Work out the finished part from the listing and answer in its coordinate system (mm). A direction names the side the tool comes from. Round coordinates to 2 decimals unless told otherwise and drop trailing zeros. Write each loop counter-clockwise with the first axis right and the second up, starting at its lowest first coordinate (ties: lowest second). Pieces come first, ordered by that corner, then holes. Notation, with made-up numbers: (48, 32) - (80, 32) arc R17 ccw to (80, 62) - close; hole circle Ø6 at (-23.75, 85). An arc over 180 degrees is marked (long way). Write item = value, one per line. Start each with the question number.
Autodesk Inventor part; units mm, degrees
ref_plane "YZ Plane" through (0, 0, 0) normal (1, 0, 0) x (0, 1, 0)
ref_plane "XZ Plane" through (0, 0, 0) normal (0, 1, 0) x (-1, 0, 0)
ref_plane "XY Plane" through (0, 0, 0) normal (0, 0, 1) x (1, 0, 0)
sketch "Skizze1" plane through (0, 0, 0) normal (0, 0, 1) x (1, 0, 0)
  line L0 (5, 52.5) -> (-5, 52.5)
  line L1 (-5, 52.5) -> (-5, 16)
  line L2 (5, 16) -> (5, 52.5)
  arc A0 (-7.9412, 4.2353) -> (7.9412, 4.2353) centre (0, 0) ccw
  arc A1 (5, 16) -> (7.9412, 4.2353) centre (30, 16) ccw
  arc A2 (-7.9412, 4.2353) -> (-5, 16) centre (-30, 16) ccw
  line L3 (0, -25.0931) -> (0, 22.9698)
  line L4 (0, 68.0186) -> (0, -40.6118)
  point P0 (0, 0)
  point P1 (0, 0)
  point P2 (-5, 7.4833)
  point P3 (5, 7.4833)
  dimension "d1" = 18
  dimension "d4" = 25
  dimension "d7" = 0
  dimension "d8" = 52.5
  dimension "d9" = 0
  dimension "d10" = 0
  dimension "d20" = 5
  dimension "d21" = 5
extrude "Extrusion1" add sketch "Skizze1" along normal blind 10
sketch "Skizze4" plane through (0, 0, 10) normal (0, 0, 1) x (1, 0, 0)
  circle A0 centre (0, 0) radius 6.05
  dimension "d22" = 12.1
extrude "Extrusion2" cut sketch "Skizze4" against normal blind 5.6
fillet "Rundung1" radius 0.2 1 edges at (-6.05, 0, 10)
fillet "Rundung2" radius 0.2 10 edges at (5, 34.25, 10) (0, -9, 10) (-5.7464, 9.9366, 10) (-5, 34.25, 10) (5.7464, 9.9366, 10) (5, 34.25, 0) (0, -9, 0) (-5.7464, 9.9366, 0) (-5, 34.25, 0) (5.7464, 9.9366, 0)
sketch "Skizze5" plane through (0, 0, 0) normal (0, 0, -1) x (-1, 0, 0)
  circle A0 centre (0, 0) radius 1.75
  dimension "d27" = 3.5
extrude "Extrusion3" cut sketch "Skizze5" against normal up to next
fillet "Rundung3" radius 0.2 2 edges at (1.75, 0, 0) (1.75, 0, 4.4)
sketch "Skizze6" plane through (-4.8, 52.5, 0) normal (0, 1, 0) x (1, 0, 0)
  circle A0 centre (4.8, -5) radius 1.75
  line L0 (9.6, -10) -> (0, -10)
  line L1 (9.8, -0.2) -> (9.8, -9.8)
  point P0 (4.8, 0)
  dimension "d31" = 3.5
  dimension "d32" = 5
  dimension "d33" = 5
extrude "Extrusion4" cut sketch "Skizze6" against normal blind 4
sketch "Skizze7" plane through (0, 0, 0) normal (0, 0, -1) x (-1, 0, 0)
  circle A0 centre (0, 0) radius 4
  dimension "d36" = 8
extrude "Extrusion5" cut sketch "Skizze7" against normal blind 3
sketch "Skizze8" plane through (0, 0, 0) normal (0, 0, -1) x (-1, 0, 0)
  line L0 (0, -13.3377) -> (18.2323, -13.3377)
  line L1 (18.2323, -13.3377) -> (18.2323, 56.3283)
  line L2 (18.2323, 56.3283) -> (0, 56.3283)
  line L3 (0, 56.3283) -> (0, -13.3377)
  point P0 (0, 0)
extrude "Extrusion6" cut sketch "Skizze8" against normal up to next
properties part number "alternativeJoint2"
1. Find section D-D on y = 22.5. Give the vertices of the cut face in (x, z), plus the area to 3 significant figures.
2. Find section C-C on z = 5. Give the vertices of the cut face in (x, y).
3. Consider line 1 (Z direction, x = 2, y = 1); line 2 (Y direction, x = 4.25, z = 8.75); line 3 (X direction, y = 21, z = 8). Determine where each line is inside the solid, lowest interval first.
4. Which of the six approach directions +Z, -Z, +X, -X, +Y, -Y give full straight-line access (tool end or side, diameter ignored) to faces 1 (the face through (1, 48.5, 5)), 2 (the face through (3, 22, 10)), 3 (the face through (5.77, 9.85, 4.93)), 4 (the face through (6.05, -0.13, 7.14)), 5 (the face through (4, 0, 1))?
5. Each of these flat-tipped pins is pushed along its axis until it touches: pin 1 (0.5 mm diameter, centred on x = 1, z = 4.5, fed in from +Y); pin 2 (1.8 mm diameter, centred on x = 4, y = 2.5, fed in from +Z). Where does it stop, or does it pass through?
6. Find section B-B on z = 1.5. Give the vertices of the cut face in (x, y).
7. For a pull along Y with two mould halves and no side action, classify faces 6 (the face through (3, 52.5, 5)), 7 (the face through (1.75, 0.04, 3.59)), 8 (the face through (5, 34, 5)) as released by +Y, released by -Y, zero draft, split by the parting line, or undercut.
8. Find section A-A on y = 0. Give the vertices of the cut face in (x, z).
Answer key:
q1.outline = (0, 0) - (4.8, 0) arc R0.2 ccw to (5, 0.2) - (5, 9.8) arc R0.2 ccw to (4.8, 10) - (0, 10) - close
q1.area = 50.0 mm²
q2.outline = (0, -9) arc R9 ccw to (7.94, 4.24) arc R25 cw to (5, 16) - (5, 52.5) - (1.75, 52.5) - (1.75, 48.5) - (0, 48.5) - (0, 6.05) arc R6.05 cw to (0, -6.05) - close
q3.line_1 = 3 to 4.4
q3.line_2 = -7.93 to -4.31, 4.31 to 52.5
q3.line_3 = 0 to 5
q4.face_1 = -X, +Y
q4.face_2 = +Z, +X, -X, +Y, -Y
q4.face_3 = +Z, -Z, +X, +Y
q4.face_4 = +Z, -X
q4.face_5 = -Z, -X
q5.pin_1 = 48.5
q5.pin_2 = 4.4
q6.outline = (0, -9) arc R9 ccw to (7.94, 4.24) arc R25 cw to (5, 16) - (5, 52.5) - (0, 52.5) - (0, 4) arc R4 cw to (0, -4) - close
q7.face_6 = released by +Y
q7.face_7 = undercut
q7.face_8 = zero draft
q8.outline = (1.75, 3) - (4, 3) - (4, 0) - (8.8, 0) arc R0.2 ccw to (9, 0.2) - (9, 9.8) arc R0.2 ccw to (8.8, 10) - (6.25, 10) arc R0.2 ccw to (6.05, 9.8) - (6.05, 4.4) - (1.95, 4.4) arc R0.2 ccw to (1.75, 4.2) - close
